from build123d import *

# Parameters (mm, degrees)
SKETCH_1_R      = 30
EXTRUDE_1_DEPTH = 1.6
EXTRUDE_2_DEPTH = 3
SKETCH_3_W      = 3.244311069
SKETCH_3_H      = 35.273993815
EXTRUDE_5_DEPTH = 1.6


with BuildPart() as part:
    # Эскиз1 → Бобышка-Вытянуть1 (new body)
    with BuildSketch(Plane(origin=(0, 0, 0), x_dir=(1, 0, 0), z_dir=(0, 1, 0))):
        Circle(SKETCH_1_R)
    extrude(amount=EXTRUDE_1_DEPTH)

    # Эскиз2 → Бобышка-Вытянуть2 (add)
    with BuildSketch(Plane(origin=(0, 1.6, 0), x_dir=(1, 0, 0), z_dir=(0, 1, 0))):
        Polygon((-15.112940101, -15.010744766), (-13.103354207, -5.79113923), (-27.098427297, -5.79113923), (-26.176466744, -1.195742096), (-6.815295119, 20.484736546), (-3.156264172, 20.484736546), (-7.974948628, -1.642316739), (-3.127452905, -1.642316739), (-4.049413459, -5.79113923), (-8.875300731, -5.79113923), (-10.884886625, -15.010744766), align=None)
        Polygon((-12.203002104, -1.642316739), (-9.112993686, 12.561638039), (-21.797154114, -1.642316739), align=None, mode=Mode.SUBTRACT)
        with BuildLine():
            Line((1.021369586, -6.713099784), (5.155786443, -6.252119507))
            add(Edge.make_bspline(
                [(5.155786443, -6.252119507), (5.192135281, -6.473381577), (5.262387165, -6.901017726), (5.397879979, -7.515231953), (5.562416953, -8.078982569), (5.75783084, -8.594252788), (5.978056496, -9.060074627), (6.225780557, -9.477912909), (6.498384414, -9.845044122), (6.888403904, -10.266320667), (7.442457962, -10.681510063), (8.162107094, -11.060328313), (8.950693699, -11.283404951), (9.495307412, -11.309570842), (9.772792028, -11.322902552)],
                knots=[0, 0, 0, 0, 0.000672606, 0.001299954, 0.00188569, 0.002432819, 0.002951522, 0.003429575, 0.003887676, 0.004320864, 0.005147809, 0.005949945, 0.006750366, 0.007581816, 0.007581816, 0.007581816, 0.007581816], degree=3))
            add(Edge.make_bspline(
                [(9.772792028, -11.322902552), (9.974836791, -11.315289739), (10.378983376, -11.300061965), (10.979375815, -11.198014835), (11.565207937, -11.022197171), (12.140680484, -10.782461737), (12.704801504, -10.469434648), (13.257512824, -10.085992109), (13.800962323, -9.638904949), (14.138144983, -9.299567127), (14.310566627, -9.12604342)],
                knots=[0, 0, 0, 0, 0.000606108, 0.001212386, 0.001820886, 0.002437558, 0.003079094, 0.003752394, 0.004453291, 0.005186777, 0.005186777, 0.005186777, 0.005186777], degree=3))
            add(Edge.make_bspline(
                [(14.310566627, -9.12604342), (14.562332157, -8.846489735), (15.074816945, -8.277440386), (15.771928843, -7.338032377), (16.413643396, -6.306492), (17.009949904, -5.193403292), (17.552241758, -3.989577112), (18.036311249, -2.697590667), (18.489551109, -1.323270245), (18.731729262, -0.366685376), (18.855544044, 0.122373383)],
                knots=[0, 0, 0, 0, 0.001128178, 0.002296479, 0.003503568, 0.004769995, 0.006082035, 0.007461238, 0.008907642, 0.010420662, 0.010420662, 0.010420662, 0.010420662], degree=3))
            add(Edge.make_bspline(
                [(18.855544044, 0.122373383), (18.515554142, -0.181681505), (17.868313732, -0.760512257), (16.895223997, -1.523524974), (15.986257834, -2.159743633), (15.121792782, -2.661558355), (14.274538335, -3.030078632), (13.434324295, -3.290513005), (12.583841099, -3.459331039), (12.011241698, -3.477265014), (11.724755387, -3.486237846)],
                knots=[0, 0, 0, 0, 0.001368042, 0.002604349, 0.003707227, 0.004694433, 0.005597662, 0.0064725, 0.007329998, 0.008188615, 0.008188615, 0.008188615, 0.008188615], degree=3))
            add(Edge.make_bspline(
                [(11.724755387, -3.486237846), (11.467545037, -3.478838371), (10.95835582, -3.464189922), (10.202997804, -3.361403617), (9.470361257, -3.188438097), (8.755779823, -2.949020303), (8.065155466, -2.63719131), (7.391074846, -2.26158419), (6.74101139, -1.813836573), (6.334287268, -1.470552033), (6.128166715, -1.296581532)],
                knots=[0, 0, 0, 0, 0.000771542, 0.001527392, 0.002282143, 0.003026964, 0.003784631, 0.004552094, 0.00533928, 0.006148115, 0.006148115, 0.006148115, 0.006148115], degree=3))
            add(Edge.make_bspline(
                [(6.128166715, -1.296581532), (5.866741871, -1.053430833), (5.344675784, -0.567858261), (4.68598861, 0.277826316), (4.120100969, 1.190125333), (3.651772278, 2.178943205), (3.306695947, 3.251277107), (3.042972026, 4.394926248), (2.892902816, 5.618933407), (2.874665369, 6.460451788), (2.865290693, 6.893021198)],
                knots=[0, 0, 0, 0, 0.001069612, 0.002136018, 0.003203397, 0.004286026, 0.00540895, 0.006576162, 0.0078028, 0.009100287, 0.009100287, 0.009100287, 0.009100287], degree=3))
            add(Edge.make_bspline(
                [(2.865290693, 6.893021198), (2.875207181, 7.388228075), (2.89472349, 8.362828189), (3.083578082, 9.796121672), (3.373185787, 11.176809481), (3.796125522, 12.501570161), (4.330630954, 13.774732447), (4.980823191, 14.99643932), (5.751264631, 16.165307898), (6.355998775, 16.881862763), (6.66117516, 17.243468975)],
                knots=[0, 0, 0, 0, 0.001484899, 0.00292238, 0.004329457, 0.005712191, 0.007087382, 0.00846651, 0.00985891, 0.011277426, 0.011277426, 0.011277426, 0.011277426], degree=3))
            add(Edge.make_bspline(
                [(6.66117516, 17.243468975), (6.934144804, 17.537158668), (7.47161345, 18.115424437), (8.359517632, 18.87278791), (9.296948211, 19.509609385), (10.272237605, 20.044447486), (11.302446737, 20.446715103), (12.37692951, 20.736367773), (13.497965187, 20.913646613), (14.261903613, 20.934929686), (14.649099018, 20.945716823)],
                knots=[0, 0, 0, 0, 0.001202159, 0.002367012, 0.003491782, 0.004597221, 0.005696684, 0.006800948, 0.007930689, 0.009091773, 0.009091773, 0.009091773, 0.009091773], degree=3))
            add(Edge.make_bspline(
                [(14.649099018, 20.945716823), (14.997787132, 20.936379292), (15.681760043, 20.918063159), (16.687233548, 20.762950374), (17.64616698, 20.504084004), (18.560197693, 20.142451509), (19.424142306, 19.676277717), (20.242163935, 19.110195911), (21.017638488, 18.442114073), (21.740577275, 17.67553899), (22.398010202, 16.814571371), (22.978272504, 15.868653702), (23.458966364, 14.829820422), (23.856664916, 13.711476165), (24.153976582, 12.506286792), (24.379655281, 11.221838923), (24.507641015, 9.848780448), (24.523306789, 8.905267443), (24.531363702, 8.420018365)],
                knots=[0, 0, 0, 0, 0.001045625, 0.002051056, 0.003043504, 0.004019904, 0.004993138, 0.00598213, 0.006998544, 0.008058362, 0.009137391, 0.010242994, 0.011380446, 0.012565085, 0.01379843, 0.015099829, 0.016474492, 0.017930103, 0.017930103, 0.017930103, 0.017930103], degree=3))
            add(Edge.make_bspline(
                [(24.531363702, 8.420018365), (24.525664072, 7.934918015), (24.514284046, 6.966354111), (24.427262909, 5.516930729), (24.273582197, 4.073215956), (24.065445524, 2.633838437), (23.799008275, 1.199214086), (23.472015699, -0.229682915), (23.095999668, -1.657124653), (22.790400156, -2.596840611), (22.637022877, -3.068474471)],
                knots=[0, 0, 0, 0, 0.001455254, 0.002905598, 0.004354081, 0.005809709, 0.007267635, 0.008730162, 0.010206528, 0.011694097, 0.011694097, 0.011694097, 0.011694097], degree=3))
            add(Edge.make_bspline(
                [(22.637022877, -3.068474471), (22.445421429, -3.608260191), (22.072409742, -4.659120639), (21.438427503, -6.164879435), (20.744443812, -7.554296537), (20.013593824, -8.845074722), (19.218836128, -10.01903208), (18.382278177, -11.090308185), (17.500898079, -12.058312556), (16.853999376, -12.618129566), (16.536237026, -12.893116619)],
                knots=[0, 0, 0, 0, 0.00171814, 0.003344892, 0.004897513, 0.006375197, 0.00779159, 0.009146026, 0.01045087, 0.011710621, 0.011710621, 0.011710621, 0.011710621], degree=3))
            add(Edge.make_bspline(
                [(16.536237026, -12.893116619), (16.275517551, -13.099437091), (15.75979639, -13.50755326), (14.936658101, -14.031619265), (14.08857004, -14.475834427), (13.213812191, -14.833383605), (12.320192974, -15.126680855), (11.398582261, -15.328844612), (10.452772335, -15.443440865), (9.813908073, -15.462246084), (9.491882172, -15.471725043)],
                knots=[0, 0, 0, 0, 0.000996907, 0.001971952, 0.002922341, 0.00386536, 0.00480383, 0.005740556, 0.006691137, 0.007657281, 0.007657281, 0.007657281, 0.007657281], degree=3))
            add(Edge.make_bspline(
                [(9.491882172, -15.471725043), (9.198617884, -15.465062279), (8.622044237, -15.451962922), (7.778171618, -15.341349076), (6.974083778, -15.163734203), (6.214126437, -14.906579258), (5.487258858, -14.594261932), (4.811253582, -14.191925812), (4.168798029, -13.730625352), (3.581420174, -13.187339966), (3.039567521, -12.584738429), (2.563524473, -11.915474189), (2.143250657, -11.193544766), (1.789964119, -10.411188257), (1.502466787, -9.568624311), (1.27386085, -8.670395225), (1.104806925, -7.712140535), (1.049695435, -7.052260618), (1.021369586, -6.713099784)],
                knots=[0, 0, 0, 0, 0.000879481, 0.001729108, 0.002548648, 0.003345854, 0.004132776, 0.004917222, 0.005700974, 0.006501394, 0.007312503, 0.008128045, 0.008960711, 0.009814936, 0.010698742, 0.011628129, 0.012593226, 0.013613817, 0.013613817, 0.013613817, 0.013613817], degree=3))
        make_face()
        with BuildLine():
            add(Edge.make_bspline(
                [(7.014113184, 7.498057811), (7.019768123, 7.243317269), (7.030786271, 6.746977844), (7.112971363, 6.022465552), (7.237466445, 5.336389944), (7.429107785, 4.691874289), (7.662640551, 4.083140966), (7.963120255, 3.518815935), (8.307660253, 2.991004091), (8.703683128, 2.507822029), (9.141020711, 2.081613788), (9.598578365, 1.703117561), (10.071970051, 1.374977493), (10.574224084, 1.115081458), (11.093650898, 0.91285426), (11.631959273, 0.767655698), (12.189958182, 0.678560926), (12.569555519, 0.667958611), (12.76196101, 0.662584645)],
                knots=[0, 0, 0, 0, 0.000764042, 0.001488668, 0.00218511, 0.002852956, 0.003503007, 0.004137714, 0.004767003, 0.005391367, 0.00600766, 0.006596047, 0.007171417, 0.007731988, 0.008288426, 0.008840559, 0.00940187, 0.009978815, 0.009978815, 0.009978815, 0.009978815], degree=3))
            add(Edge.make_bspline(
                [(12.76196101, 0.662584645), (13.05139438, 0.676731012), (13.638138298, 0.705408752), (14.512398022, 0.935715715), (15.382277568, 1.299423228), (16.240003107, 1.808003519), (17.070741272, 2.454050946), (17.83396819, 3.259410645), (18.547032162, 4.195807232), (19.170277098, 5.263560877), (19.709790373, 6.398811887), (20.094032745, 7.57986936), (20.33518312, 8.775140421), (20.366777551, 9.580970443), (20.382541211, 9.983029616)],
                knots=[0, 0, 0, 0, 0.000867334, 0.001758273, 0.002694639, 0.003689072, 0.004740905, 0.005841216, 0.007008095, 0.008264383, 0.009543689, 0.010771405, 0.011982014, 0.013187491, 0.013187491, 0.013187491, 0.013187491], degree=3))
            add(Edge.make_bspline(
                [(20.382541211, 9.983029616), (20.372951463, 10.295722068), (20.354025111, 10.912852788), (20.200419667, 11.820980608), (19.936709411, 12.688869248), (19.587274972, 13.514264205), (19.151964964, 14.277348135), (18.633780293, 14.952051568), (18.035571041, 15.522736313), (17.372002119, 15.97945588), (16.675354278, 16.338724835), (15.964465751, 16.60024492), (15.24524014, 16.769356322), (14.760441115, 16.787750578), (14.519448315, 16.796894332)],
                knots=[0, 0, 0, 0, 0.000937723, 0.001850692, 0.002753088, 0.003653468, 0.004534364, 0.005381515, 0.006196675, 0.007003905, 0.007789937, 0.008541933, 0.009272406, 0.009994451, 0.009994451, 0.009994451, 0.009994451], degree=3))
            add(Edge.make_bspline(
                [(14.519448315, 16.796894332), (14.288282748, 16.789085648), (13.824283604, 16.773411934), (13.13177034, 16.628464349), (12.446585191, 16.395690831), (11.768928129, 16.078840648), (11.110004943, 15.671818458), (10.476966926, 15.17730675), (9.858820739, 14.606825776), (9.28343841, 13.947489545), (8.752685138, 13.222672572), (8.278203551, 12.443585563), (7.892711178, 11.60155963), (7.576689262, 10.730159546), (7.323697649, 9.861582737), (7.155792922, 9.02703603), (7.036547924, 8.245734242), (7.02140133, 7.740947846), (7.014113184, 7.498057811)],
                knots=[0, 0, 0, 0, 0.00069282, 0.001390638, 0.002112683, 0.00286025, 0.003629874, 0.00443091, 0.005266747, 0.006149643, 0.007051492, 0.007959419, 0.008881042, 0.009824418, 0.010738609, 0.011591831, 0.012377202, 0.013105578, 0.013105578, 0.013105578, 0.013105578], degree=3))
        make_face(mode=Mode.SUBTRACT)
    extrude(amount=EXTRUDE_2_DEPTH)

    # Эскиз3 → Бобышка-Вытянуть5 (add)
    with BuildSketch(Plane.XZ):
        with Locations((0.764892295, 38.487099642)):
            Rectangle(SKETCH_3_W, SKETCH_3_H)
    extrude(amount=-EXTRUDE_5_DEPTH)


solid = part.part
The listing builds one solid part. Answer for the finished solid, in the listing's coordinates (mm). A direction names the side the tool comes from. Give positions to 0.01 mm unless a question says otherwise; leave off trailing zeros. Order: outer loops, then holes, each group sorted by start corner. A loop starts at its lowest first (then second) coordinate and runs counter-clockwise, first axis right, second up. Notation, with made-up numbers: (21.5, 66) - (46.5, 66) arc R10 ccw to (46.5, 84) - close; hole circle Ø6 at (6, 50.25). An arc over 180 degrees is marked (long way). Use one line per item in the form item = value.
1) Consider probe 1 along X at (y, z) = (1.75, -8); probe 2 along Z at (x, y) = (12, 1.7); probe 3 along Y at (x, z) = (11, -14). Determine where each line is inside the solid, lowest interval first. Write a range as [from, to].
Verdict:
probe_1 = [-17.96, -13.19], [-10.11, -5.88], [2.9, 7.03], [20.17, 24.53]
probe_2 = [-20.63, -16.18], [-0.71, 3.48], [10.84, 15.19]
probe_3 = [0, 1.6]
2) Find section C-C on z = 47.5. Determine the outline of the cut face in (x, y).
Verdict:
outline = (-0.86, 0) - (2.39, 0) - (2.39, 1.6) - (-0.86, 1.6) - close
3) Each of these flat-tipped pins is pushed along its axis until it touches: pin 1 (0.8 mm diameter, centred on y = 0.5, z = 45.5, fed in from +X); pin 2 (18 mm diameter, centred on x = 7.5, z = 30, fed in from +Y); pin 3 (5 mm diameter, centred on x = -6.5, z = -2.5, fed in from -Y); pin 4 (1.5 mm diameter, centred on x = -6.5, y = 3.5, fed in from +Z). Where does it stop, or does it pass through?
Verdict:
pin_1 = 2.39
pin_2 = 1.6
pin_3 = 0
pin_4 = 5.79
4) The mould has two halves that part along Z. Classify faces 1 (the flat face through (-5, 3, -20.485)), 2 (the flat face through (-9.866, 3.079, 10.336)), 3 (the flat face through (-17, 3, 1.642)): released by +Z, released by -Z, zero draft, split by the parting line, or undercut.
Verdict:
face_1 = released by -Z
face_2 = released by +Z
face_3 = undercut
5) Find section B-B on x = 0. Determine the outline of the cut face in (y, z).
Verdict:
outline = (0, -30) - (1.6, -30) - (1.6, 56.12) - (0, 56.12) - close
6) For faces 4 (the flat face through (-16.631, 3.079, -9.493)), 5 (the flat face through (-15.366, 3.079, -5.559)), 6 (the flat face through (-13, 3, 15.011)), 7 (the flat face through (-6, 3, 5.791)), 8 (the flat face through (-0.857, 1, 43)), determine the directions among +Z, -Z, +X, -X, +Y, -Y from which every point of the face is accessible in a straight line to the end or side of a thin tool.
Verdict:
face_4 = -Z, -X, +Y
face_5 = +Y
face_6 = +Z, -X, +Y
face_7 = +Z, +Y
face_8 = +Z, -X, +Y, -Y
7) Find section A-A on y = 3.45. Give the number of separate pieces and of enclosed holes in the cut face, and give its area (3 significant figures).
Verdict:
separate_pieces = 2
enclosed_holes = 2
area = 695 mm^2
